Can you work these out from the drawing? Everything is in mm from the part's minimum corner. A direction names the side the tool comes from. Give positions to 0.01 mm unless a question says otherwise; leave off trailing zeros. Order: outer loops, then holes, each group sorted by start corner. A loop starts at its lowest first (then second) coordinate and runs counter-clockwise, first axis right, second up. Notation, with made-up numbers: (-31, 41) - (-6, 41) arc R22 ccw to (-6, 69) - close; hole circle Ø1 at (61, -21). An arc over 180 degrees is marked (long way). One line per question, with ' | ' between items.
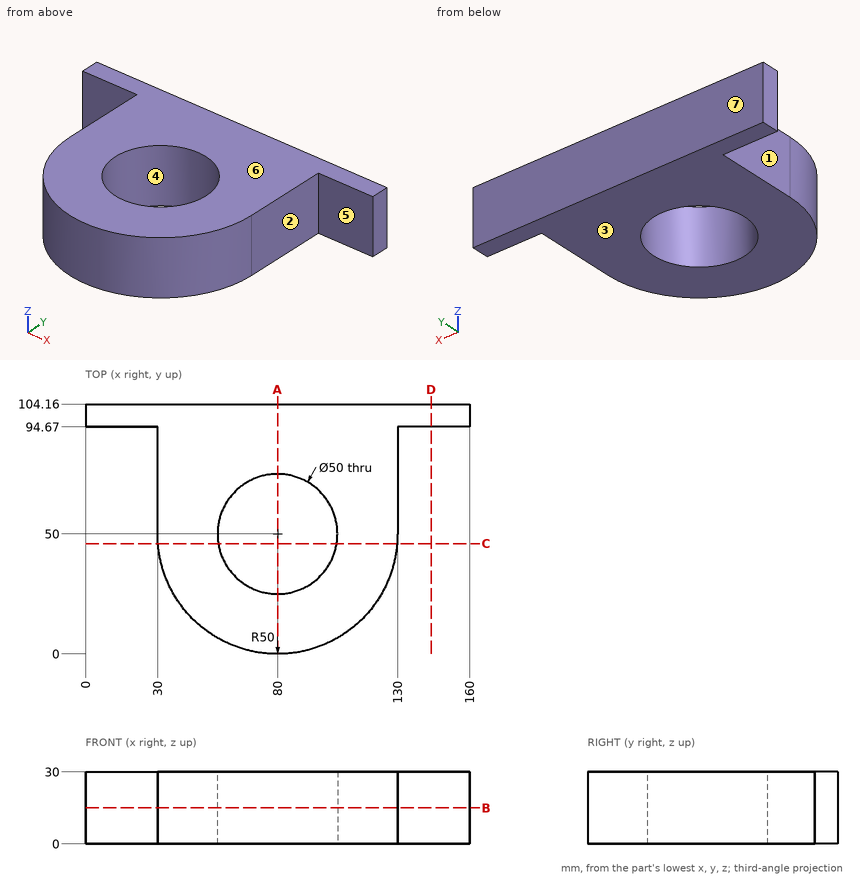
1) I want a section at D-D (x = 144). List the corners of the cut face in (y, z) for me, plus the area to 3 significant figures.
Model answer:
outline: (94.67, 0) - (104.16, 0) - (104.16, 30) - (94.67, 30) - close | area: 285 mm2
2) Thinking about a two-plate mould opening in Y: for the marked faces 4, 5, 6 and 7, which applies, +Y half, -Y half, draft (parallel to the pull), parting line (faces both ways), or undercut?
Model answer:
face 4: undercut | face 5: -Y half | face 6: draft | face 7: +Y half
3) I want a section at B-B (z = 15). List the corners of the cut face in (x, y) for me.
Model answer:
outline: (0, 94.67) - (30, 94.67) - (30, 50) arc R50 ccw to (130, 50) - (130, 94.67) - (160, 94.67) - (160, 104.16) - (0, 104.16) - close; hole circle Ø50 at (80, 50)
4) Please list where these lines run through material, in increasing order: L1, parallel to Y at x = 80, z = 10.5; L2, parallel to Y at x = 9.5, z = 14.25; L3, parallel to Y at x = 93, z = 14.25.
Model answer:
L1: y = 0 to 25, 75 to 104.16 | L2: y = 94.67 to 104.16 | L3: y = 1.72 to 28.65, 71.35 to 104.16
5) On a 3-axis mill with a long thin cutter (end or side, diameter ignored), from which of +Z, -Z, +X, -X, +Y, -Y can I reach the whole of each face in a straight line? I mean the marked faces 1, 2 and 3. Say none if no direction works.
Model answer:
face 1: +Z, -Z, -X, -Y | face 2: +Z, -Z, +X, -Y | face 3: -Z, +X, -X, +Y, -Y
6) I want a section at A-A (x = 80). List the corners of the cut face in (y, z) for me, plus the area to 3 significant figures.
Model answer:
outline: (0, 0) - (25, 0) - (25, 30) - (0, 30) - close; (75, 0) - (104.16, 0) - (104.16, 30) - (75, 30) - close | area: 1,620 mm2
7) I'm going to push flat-ended pins straight in: P1, Ø2, axis at y = 87, z = 17, coming from the -X side; P2, Ø12, axis at y = 67, z = 21.5, coming from the +X side; P3, Ø1, axis at x = 140.5, z = 4, coming from the -Y side. Where does each tip first touch, or does it pass through?
Model answer:
P1: stops at x = 30 | P2: stops at x = 130 | P3: stops at y = 94.67
8) I want a section at C-C (y = 46). List the corners of the cut face in (x, z) for me.
Model answer:
outline: (30.16, 0) - (55.32, 0) - (55.32, 30) - (30.16, 30) - close; (104.68, 0) - (129.84, 0) - (129.84, 30) - (104.68, 30) - close
